Work out the finished part from the listing and answer in its coordinate system (mm). A direction names the side the tool comes from. Coordinates: 2 decimals unless noted, no trailing zeros. Order: outer loops, then holes, each group sorted by start corner. A loop starts at its lowest first (then second) coordinate and runs counter-clockwise, first axis right, second up. Notation, with made-up numbers: M 62,55.5 L 73,55.5 A20 ccw 73,85.5 Z; hole C 26.25,-5 d6. An arc over 180 degrees is marked long. Use a Markdown table: item, result.
from build123d import *

# Parameters (mm, degrees)
CUT_EXTRUDE1_DEPTH           = 25
CUT_EXTRUDE1_DEPTH_BACK      = 25
CUT_EXTRUDE2_DEPTH           = 25
CUT_EXTRUDE2_DEPTH_BACK      = 25
CUT_EXTRUDE3_DEPTH           = 25
CUT_EXTRUDE3_DEPTH_BACK      = 25
SKETCH5_W                    = 31.1
SKETCH5_H                    = 6
CUT_REVOLVE3_ANGLE           = 90
CUT_REVOLVE3_OTHER_WAY_ANGLE = 90


with BuildPart() as part:
    # Sketch1 → Revolve1 (revolve)
    with BuildSketch(Plane(origin=(0, 0, 0), x_dir=(0, 0, -1), z_dir=(1, 0, 0))):
        with BuildLine():
            Line((-14, 0), (-14, 24))
            Line((-14, 24), (26.650635095, 24))
            Line((26.650635095, 24), (30, 11.5))
            ThreePointArc((30, 11.5), (30.439339828, 10.439339828), (31.5, 10))
            Line((31.5, 10), (47, 10))
            ThreePointArc((47, 10), (47.707106781, 9.707106781), (48, 9))
            Line((48, 9), (48, 0))
            Line((48, 0), (-14, 0))
        make_face()
    revolve(axis=Axis((0, 0, -48), (0, 0, 1)))

    # Sketch2 → Cut-Extrude1 (cut, two sides)
    with BuildSketch(Plane(origin=(0, 0, 0), x_dir=(1, 0, 0), z_dir=(0, 1, 0))) as cut_extrude1_sk:
        Polygon((-6, 23), (-6, -15), (6, -15), (6, 23), (5, 24), (-5, 24), align=None)
    extrude(amount=CUT_EXTRUDE1_DEPTH, mode=Mode.SUBTRACT)
    extrude(cut_extrude1_sk.sketch, amount=-CUT_EXTRUDE1_DEPTH_BACK, mode=Mode.SUBTRACT)

    # Sketch3 → Cut-Extrude2 (cut, two sides)
    with BuildSketch(Plane(origin=(0, 0, 0), x_dir=(0, 0, -1), z_dir=(1, 0, 0))) as cut_extrude2_sk:
        Polygon((-39, -36), (48, -36), (48, -12), (-15, -12), (-15, 12), (48, 12), (48, 36), (-39, 36), align=None)
    extrude(amount=CUT_EXTRUDE2_DEPTH, mode=Mode.SUBTRACT)
    extrude(cut_extrude2_sk.sketch, amount=-CUT_EXTRUDE2_DEPTH_BACK, mode=Mode.SUBTRACT)

    # Sketch4 → Cut-Extrude3 (cut, two sides)
    with BuildSketch(Plane(origin=(0, 0, 0), x_dir=(1, 0, 0), z_dir=(0, 1, 0))) as cut_extrude3_sk:
        Polygon((-36, -39), (36, -39), (36, 48), (12, 48), (12, -15), (-12, -15), (-12, 48), (-36, 48), align=None)
    extrude(amount=CUT_EXTRUDE3_DEPTH, mode=Mode.SUBTRACT)
    extrude(cut_extrude3_sk.sketch, amount=-CUT_EXTRUDE3_DEPTH_BACK, mode=Mode.SUBTRACT)

    # Sketch5 → Cut-Revolve1 (revolve, cut)
    with BuildSketch(Plane.XY):
        with Locations((0, 3)):
            Rectangle(SKETCH5_W, SKETCH5_H)
    revolve(axis=Axis((15.55, 0, 0), (-1, 0, 0)), mode=Mode.SUBTRACT)

    # Sketch6 → Cut-Revolve2 (revolve, cut)
    with BuildSketch(Plane(origin=(0, 0, 0), x_dir=(0, 0, -1), z_dir=(1, 0, 0))):
        Polygon((22.9, 0), (22.9, 5.053), (47.153, 5.053), (48.1, 6), (48.1, 0), align=None)
    revolve(axis=Axis((0, 0, -48.1), (0, 0, 1)), mode=Mode.SUBTRACT)

    # Sketch7 → Cut-Revolve3 (revolve, cut)
    with BuildSketch(Plane(origin=(0, 0, 0), x_dir=(1, 0, 0), z_dir=(0, 1, 0))):
        Polygon((-14, -9.42346282), (-14, -37.136275741), (0, -45.219179509), (14, -37.136275741), (14, -9.42346282), (0, -17.506366588), align=None)
    revolve(axis=Axis((-14, 0, -24), (1, 0, 0)), revolution_arc=CUT_REVOLVE3_ANGLE, mode=Mode.SUBTRACT)

    # Sketch7 → Cut-Revolve3 other way (revolve, cut)
    with BuildSketch(Plane(origin=(0, 0, 0), x_dir=(1, 0, 0), z_dir=(0, 1, 0))):
        Polygon((-14, -9.42346282), (-14, -37.136275741), (0, -45.219179509), (14, -37.136275741), (14, -9.42346282), (0, -17.506366588), align=None)
    revolve(axis=Axis((-14, 0, -24), (-1, 0, 0)), revolution_arc=CUT_REVOLVE3_OTHER_WAY_ANGLE, mode=Mode.SUBTRACT)


solid = part.part
1. For faces 1 (the face through (9.76, -2.17, -39.36)), 2 (the face through (-6, 0, -9)), 3 (the face through (3.075, -4.01, -35.707)), determine the directions among +Z, -Z, +X, -X, +Y, -Y from which every point of the face is accessible in a straight line to the end or side of a thin tool.
Answers below:
| item | result |
|---|---|
| face 1 | -Z |
| face 2 | +Z, +Y, -Y |
| face 3 | +Z, -Z |
2. For a pull along Z with two mould halves and no side action, classify faces 4 (the face through (-9, -6, 0)), 5 (the face through (-12, 0, -9)), 6 (the face through (-9.042, 0.18, 12.286)), 7 (the face through (9, -6, 0)) as +Z half, -Z half, draft (parallel to the pull), parting line (faces both ways), or undercut.
Answers below:
| item | result |
|---|---|
| face 4 | undercut |
| face 5 | draft |
| face 6 | +Z half |
| face 7 | undercut |
3. Section A-A on z = 0 is taken. Determine the outline of the cut face in (x, y), then the cut area to 3 significant figures.
Answers below:
| item | result |
|---|---|
| outline | M -12,-12 L -6,-12 L -6,-6 L -12,-6 Z; M -12,6 L -6,6 L -6,12 L -12,12 Z; M 6,-12 L 12,-12 L 12,-6 L 6,-6 Z; M 6,6 L 12,6 L 12,12 L 6,12 Z |
| area | 144 mm² |
4. Flat-ended cylindrical pins translate along their axes: P1, Ø6, axis at x = 9, y = 4.5, coming from the +Z side; P2, Ø1.5, axis at y = -6, z = -35, coming from the +X side; P3, Ø1, axis at y = -3.5, z = -39.5, coming from the +X side. Find the tip coordinate at first contact, or state that the pin passes through.
Answers below:
| item | result |
|---|---|
| P1 | z = 13.81 |
| P2 | x = 8.51 |
| P3 | x = 9.54 |
5. Section B-B on x = 0 is taken. Determine the outline of the cut face in (y, z).
Answers below:
| item | result |
|---|---|
| outline | M -12,-29.87 L -11.5,-30 A1.5 cw -10,-31.5 L -10,-47 A1 ccw -9,-48 L -5.9,-48 L -5.05,-47.15 L -5.05,-24 L -12,-24 Z; M 5.05,-47.15 L 5.9,-48 L 9,-48 A1 ccw 10,-47 L 10,-31.5 A1.5 cw 11.5,-30 L 12,-29.87 L 12,-24 L 5.05,-24 Z |
6. Section D-D on y = 4 is taken. Give the number of separate pieces and of enclosed holes in the cut face, then the cut area to 3 significant figures.
Answers below:
| item | result |
|---|---|
| separate pieces | 4 |
| enclosed holes | 0 |
| area | 652 mm² |
7. Find the intervals of material crossed by probe 1 along Y at (x, z) = (0, -31.75); probe 2 along X at (y, z) = (8.5, -4.5), in increasing order.
Answers below:
| item | result |
|---|---|
| probe 1 | -10 to -5.05, 5.05 to 10 |
| probe 2 | -12 to -6, 6 to 12 |
8. Section C-C on z = -36.5 is taken. Determine the outline of the cut face in (x, y).
Answers below:
| item | result |
|---|---|
| outline | C 0,0 d20; hole C 0,0 d10.11 |
